from build123d import *

# Parameters (mm, degrees)
F1_DEPTH      = 65
F2_R          = 1.5
F3_DEPTH      = 21.001
F4_R          = 1.5
F5_DEPTH      = 21.001
F5_DEPTH_BACK = 6.001
F6_SIZE       = 2
F7_W          = 15.7
F7_H          = 15.7
F8_DEPTH      = 65.001


with BuildPart() as f1:
    # F0 (on Right) → F1 (new body)
    with BuildSketch(Plane.YZ):
        Polygon((-7.5, 7.5), (7.5, 7.5), (7.5, 13.5), (-13.5, 13.5), (-13.5, -13.5), (7.5, -13.5), (7.5, -7.5), (-7.5, -7.5), align=None)
    extrude(amount=F1_DEPTH)

    # F2 (on face) → F3 (cut, through all)
    with BuildSketch(Plane.XZ.offset(13.5)):
        with Locations((10, 0)):
            Circle(F2_R)
        with Locations((55, 0)):
            Circle(F2_R)
    extrude(amount=-F3_DEPTH, mode=Mode.SUBTRACT)

    # F4 (on face) → F5 (cut, two sides)
    with BuildSketch(Plane(origin=(0, 0, 7.5), x_dir=(1, 0, 0), z_dir=(0, 0, -1))) as f5_sk:
        with Locations((55, 0)):
            Circle(F4_R)
        with Locations((10, 0)):
            Circle(F4_R)
    extrude(amount=F5_DEPTH, mode=Mode.SUBTRACT)
    extrude(f5_sk.sketch, amount=-F5_DEPTH_BACK, mode=Mode.SUBTRACT)

    # F6
    f6_edges = [f1.edges().sort_by_distance(p)[0] for p in [
        (53.5, 0, 13.5),
        (8.5, 0, 13.5),
        (8.5, -13.5, 0),
        (53.5, -13.5, 0),
        (53.5, 0, -13.5),
        (8.5, 0, -13.5),
    ]]
    chamfer(f6_edges, length=F6_SIZE)

    # F7 (on face) → F8 (cut, through all)
    with BuildSketch(Plane(origin=(0, 0, 0), x_dir=(0, -1, 0), z_dir=(-1, 0, 0))):
        Rectangle(F7_W, F7_H)
    extrude(amount=-F8_DEPTH, mode=Mode.SUBTRACT)


solid = f1.part
The listing builds one solid part. Answer for the finished solid, in the listing's coordinates (mm). A direction names the side the tool comes from. Coordinates: 2 decimals unless noted, no trailing zeros. Write each loop counter-clockwise with the first axis right and the second up, starting at its lowest first coordinate (ties: lowest second). Pieces come first, ordered by that corner, then holes. Notation, with made-up numbers: (-6, 87.5) - (35, 87.5) arc R13 ccw to (35, 106.5) - close; hole circle Ø9 at (32, -13.5). An arc over 180 degrees is marked (long way). Answer as CSV lines item,"result".
1. Find section B-B (x = 55). Give the vertices of the cut face in (y, z).
Computed values:
outline,"(-13.5, -13.5) - (-3.5, -13.5) - (-1.5, -11.5) - (-1.5, -7.85) - (-7.85, -7.85) - (-7.85, -1.5) - (-11.5, -1.5) - (-13.5, -3.5) - close; (-13.5, 3.5) - (-11.5, 1.5) - (-7.85, 1.5) - (-7.85, 7.85) - (-1.5, 7.85) - (-1.5, 11.5) - (-3.5, 13.5) - (-13.5, 13.5) - close; (1.5, -11.5) - (3.5, -13.5) - (7.5, -13.5) - (7.5, -7.85) - (1.5, -7.85) - close; (1.5, 7.85) - (7.5, 7.85) - (7.5, 13.5) - (3.5, 13.5) - (1.5, 11.5) - close"
2. Find section A-A (z = 0). Give the vertices of the cut face in (x, y).
Computed values:
outline,"(0, -13.5) - (6.5, -13.5) - (8.5, -11.5) - (8.5, -7.85) - (0, -7.85) - close; (11.5, -11.5) - (13.5, -13.5) - (51.5, -13.5) - (53.5, -11.5) - (53.5, -7.85) - (11.5, -7.85) - close; (56.5, -11.5) - (58.5, -13.5) - (65, -13.5) - (65, -7.85) - (56.5, -7.85) - close"
3. Find section D-D (x = 28). Give the vertices of the cut face in (y, z), plus the area to 3 significant figures.
Computed values:
outline,"(-13.5, -13.5) - (7.5, -13.5) - (7.5, -7.85) - (-7.85, -7.85) - (-7.85, 7.85) - (7.5, 7.85) - (7.5, 13.5) - (-13.5, 13.5) - close"
area,"326 mm²"
4. Determine the mould class of faces 1 (the cylindrical face through (56.43, -0.45, 9.65)), 2 (the conical face through (12, 0, -12)), 3 (the flat face through (32, 0, -7.85)) for opening direction Z: +Z half, -Z half, draft (parallel to the pull), parting line (faces both ways), or undercut.
Computed values:
face 1,"draft"
face 2,"-Z half"
face 3,"undercut"
5. A tool of negligible diameter and unlimited length cuts with its end or side. For faces 4 (the flat face through (32, -3, 13.5)), 5 (the flat face through (32, 0, 7.85)), from which of +Z, -Z, +X, -X, +Y, -Y can it reach the whole face along a straight path? Write none if from no direction.
Computed values:
face 4,"+Z, +X, -X, +Y, -Y"
face 5,"+X, -X, +Y"
6. Given P1, Ø10, axis at x = 54.5, y = 1, coming from the -Z side; P2, Ø4, axis at x = 10, y = 0, coming from the -Z side; P3, Ø3.5, axis at x = 55, y = 0, coming from the +Z side; P4, Ø3.5, axis at x = 10, y = 0, coming from the -Z side, each flat-ended and moving along its own axis, determine where each tip first touches the part or whether it passes through.
Computed values:
P1,"stops at z = -13.5"
P2,"stops at z = -12"
P3,"stops at z = 11.75"
P4,"stops at z = -11.75"
7. Find section C-C (y = 0). Give the number of separate pieces and of enclosed holes in the cut face, plus the area to 3 significant figures.
Computed values:
separate pieces,"6"
enclosed holes,"0"
area,"651 mm²"
8. Straight lines are drawn through the part: line 1 (X direction, y = 0, z = 9.25); line 2 (Z direction, x = 13.5, y = 4); line 3 (Z direction, x = 55, y = -8.95). For each, find the intervals that lie inside material, in ascending order. Write a range as [from, to].
Computed values:
line 1,"x = [0, 8.5], [11.5, 53.5], [56.5, 65]"
line 2,"z = [-13.5, -7.85], [7.85, 13.5]"
line 3,"z = [-13.5, -1.5], [1.5, 13.5]"
